```python
from build123d import *

# Parameters (mm, degrees)
F1_DEPTH = 12.7
F2_R     = 50.8
F3_R     = 38.1
F4_R     = 25.39999


# Not quite as in the source:
# - a fillet or chamfer is up to 0.001 mm smaller than in the source, because OpenCascade refuses the exact size


with BuildPart() as f1:
    # F0 (on Top) → F1 (new body)
    with BuildSketch(Plane.XY):
        Polygon((-50.8, 381), (-127, 381), (-127, 0), (-127, -381), (-50.8, -381), (-50.8, -533.4), (50.8, -533.4), (50.8, -381), (127, -381), (127, 0), (127, 381), (50.8, 381), (50.8, 533.4), (-50.8, 533.4), align=None)
    extrude(amount=F1_DEPTH)

    # F2
    f2_edges = [f1.edges().sort_by_distance(p)[0] for p in [
        (-50.8, 381, 6.35),
        (50.8, 381, 6.35),
        (-50.8, -381, 6.35),
        (50.8, -381, 6.35),
    ]]
    fillet(f2_edges, radius=F2_R)

    # F3
    f3_edges = [f1.edges().sort_by_distance(p)[0] for p in [
        (-50.8, 533.4, 6.35),
        (50.8, 533.4, 6.35),
        (-50.8, -533.4, 6.35),
        (50.8, -533.4, 6.35),
    ]]
    fillet(f3_edges, radius=F3_R)

    # F4 (radius 25.4 in the source; OpenCascade refuses exactly that, so slightly less here)
    f4_edges = [f1.edges().sort_by_distance(p)[0] for p in [
        (-127, 381, 6.35),
        (127, 381, 6.35),
        (127, -381, 6.35),
        (-127, -381, 6.35),
    ]]
    fillet(f4_edges, radius=F4_R)


solid = f1.part
```
The model under review builds one solid part; all positions refer to its coordinate system, in mm. Coordinates: 2 decimals unless noted, no trailing zeros. Order: outer loops, then holes, each group sorted by start corner. A loop starts at its lowest first (then second) coordinate and runs counter-clockwise, first axis right, second up. Notation, with made-up numbers: M 54,18 L 64,18 A37 ccw 64,56 Z; hole C 62,65 d8. An arc over 180 degrees is marked long. One line per question, with ' | ' between items.
(1) For probe 1 along Y at (x, z) = (-104.5, 5.5); probe 2 along X at (y, z) = (484, 7.5); probe 3 along X at (y, z) = (407, 3.75), list the stretches that pass through material, from the lowest coordinate up. Write a range as from..to.
Geometry results:
probe 1: y = -380.83..380.83 | probe 2: x = -50.8..50.8 | probe 3: x = -57.26..57.26
(2) Add section C-C, the plane x = -69.5. Write out the cut boundary in (y, z).
Geometry results:
outline: M -392.43,0 L 392.43,0 L 392.43,12.7 L -392.43,12.7 Z
(3) Add section B-B, the plane x = 83. Write out the cut boundary in (y, z).
Geometry results:
outline: M -384.53,0 L 384.53,0 L 384.53,12.7 L -384.53,12.7 Z
(4) Insertion check: pin 1 (3 mm diameter, centred on x = 66, z = 3.5, fed in from +Y); pin 2 (4 mm diameter, centred on y = -450.5, z = 3.5, fed in from -X); pin 3 (1.5 mm diameter, centred on y = -358, z = 2, fed in from -X). Each pin has a flat end and moves straight along its axis. Give the tip position at first contact, or say it passes through.
Geometry results:
pin 1: stops at y = 397.1 | pin 2: stops at x = -50.8 | pin 3: stops at x = -126.95
